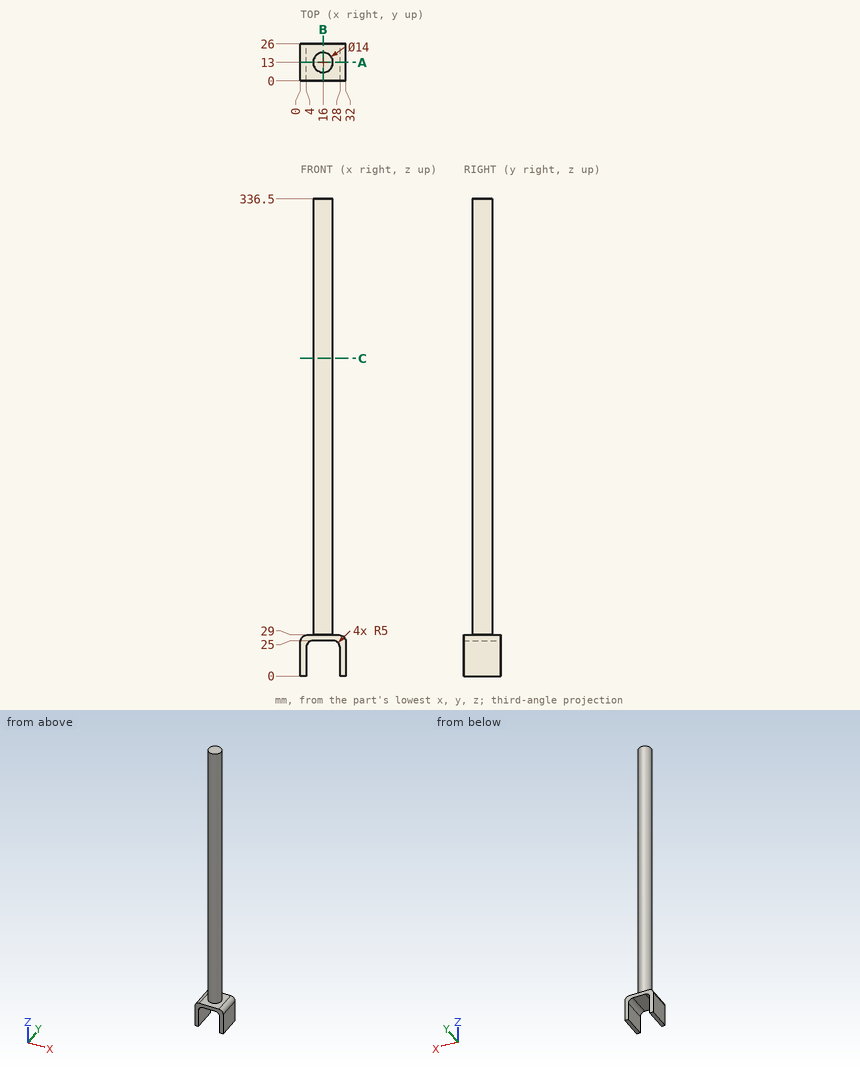
Check sheet for the drawn part. Datum: minimum x, y, z corner. Units: mm. Round coordinates to 2 decimals unless told otherwise and drop trailing zeros. Loops run counter-clockwise (first coordinate to the right, second up) from the corner with the lowest first, then second, coordinate; pieces in that order, holes last. Notation, with made-up numbers: (58, -16) - (82, -16) arc R18 cw to (82, 16) - close; hole circle Ø3 at (-20, 52.25). An arc over 180 degrees is marked (long way). Write item = value, one per line. Start each with the question number.
1. Depth check by flat-ended pin: pin 1 (6 mm diameter, centred on x = 26.5, z = 173.5, fed in from -Y); pin 2 (3 mm diameter, centred on x = 15, z = 183.5, fed in from -Y); pin 3 (15.5 mm diameter, centred on x = 17.5, y = 15, fed in from -Z); pin 4 (4 mm diameter, centred on x = 12, y = 7.5, fed in from -Z). Enter the tip coordinate at first touch or a pass-through.
2. Section check C-C on z = 224. Enter the section's corners in (x, y).
3. Thickness scan on line 1 (Z direction, x = 19, y = 17.25); line 2 (Z direction, x = 12.5, y = 6); line 3 (Y direction, x = 21, z = 83). Record the ranges inside material, lowest first.
4. Section check B-B on x = 16. Enter the section's corners in (y, z), then the cut area to 3 significant figures.
5. Section check A-A on y = 13. Enter the section's corners in (x, z), then the cut area to 3 significant figures.
Working result:
q1.pin_1 = through
q1.pin_2 = 6
q1.pin_3 = 24.47
q1.pin_4 = 25
q2.outline = circle Ø14 at (16, 13)
q3.line_1 = 25 to 336.5
q3.line_2 = 25 to 29
q3.line_3 = 8.1 to 17.9
q4.outline = (0, 25) - (26, 25) - (26, 29) - (20, 29) - (20, 336.5) - (6, 336.5) - (6, 29) - (0, 29) - close
q4.area = 4,410 mm^2
q5.outline = (0, 0) - (4, 0) - (4, 20) arc R5 cw to (9, 25) - (23, 25) arc R5 cw to (28, 20) - (28, 0) - (32, 0) - (32, 24) arc R5 ccw to (27, 29) - (23, 29) - (23, 336.5) - (9, 336.5) - (9, 29) - (5, 29) arc R5 ccw to (0, 24) - close
q5.area = 4,630 mm^2
